Check sheet for the modelled part. Datum: model origin and axes. Units: mm. A direction names the side the tool comes from. Give positions to 0.01 mm unless a question says otherwise; leave off trailing zeros. Loops run counter-clockwise (first coordinate to the right, second up) from the corner with the lowest first, then second, coordinate; pieces in that order, holes last. Notation, with made-up numbers: (-25.5, -4.5) - (-11.5, -4.5) arc R18 cw to (-11.5, 28.5) - close; hole circle Ø4 at (87.5, 11.5). An arc over 180 degrees is marked (long way). Use one line per item in the form item = value.
from build123d import *

# Parameters (mm, degrees)
F0_W     = 714.670822
F0_H     = 1041.4
F1_DEPTH = 1397
F2_DEPTH = 1143
F0_W_2   = 127
F0_H_2   = 660.4
F3_DEPTH = 1092.2
F4_W     = 596.427142
F4_H     = 931.297839
F5_DEPTH = 873.76


with BuildPart() as f1:
    # F0 (on Top) → F1 (new body)
    with BuildSketch(Plane.XY):
        with Locations((988.864589, 12.7)):
            Rectangle(F0_W, F0_H)
    extrude(amount=F1_DEPTH)

    # F0 (on Top) → F2 (join)
    with BuildSketch(Plane.XY):
        Polygon((-203.2, 0), (0, 0), (0, -508), (631.529178, -508), (631.529178, 533.4), (799.153613, 903.620216), (58.713181, 1238.869088), (-203.2, 660.4), align=None)
    extrude(amount=F2_DEPTH)

    # F0 (on Top) → F3 (join)
    with BuildSketch(Plane.XY):
        with Locations((-266.7, 330.2)):
            Rectangle(F0_W_2, F0_H_2)
    extrude(amount=F3_DEPTH)

    # F4 (on face) → F5 (cut)
    with BuildSketch(Plane.XY.offset(1397)):
        with Locations((996.125251, 10.54573)):
            Rectangle(F4_W, F4_H)
    extrude(amount=-F5_DEPTH, mode=Mode.SUBTRACT)


solid = f1.part
Item 1: Section check C-C on y = 161.5. Record the boundary of the cut face in (x, z).
Answer block:
outline = (-330.2, 0) - (1346.2, 0) - (1346.2, 1397) - (1294.34, 1397) - (1294.34, 523.24) - (697.91, 523.24) - (697.91, 1397) - (631.53, 1397) - (631.53, 1143) - (-203.2, 1143) - (-203.2, 1092.2) - (-330.2, 1092.2) - close
Item 2: Section check A-A on z = 1206. Record the boundary of the cut face in (x, y), then the cut area to 3 significant figures.
Answer block:
outline = (631.53, -508) - (1346.2, -508) - (1346.2, 533.4) - (631.53, 533.4) - close; hole (697.91, -455.1) - (1294.34, -455.1) - (1294.34, 476.19) - (697.91, 476.19) - close
area = 189,000 mm2
Item 3: Access from +Z, -Z, +X, -X, +Y, -Y to the whole of each face (thin tool, end or side, straight path). Record for faces 1 (the face through (714.17, 715.92, 563.5)), 2 (the face through (992, -455.103, 966)), 3 (the face through (0, -250, 563)), 4 (the face through (434.116, 1068.898, 563.499)), 5 (the face through (-268, 335, 1092.2)).
Answer block:
face_1 = +Z, -Z, +X
face_2 = +Z
face_3 = +Z, -Z, -X, -Y
face_4 = +Z, -Z, +X, +Y
face_5 = +Z, -X, +Y, -Y
Item 4: Gauge pin test, flat ends, axial feed: P1, Ø4, axis at x = 895.5, y = -204.5, coming from the +Z side; P2, Ø8, axis at y = 1028.5, z = 668.5, coming from the -X side; P3, Ø2, axis at y = -60.5, z = 962, coming from the -X side. Record the tip position at first contact, or that the pin passes through.
Answer block:
P1 = 523.24
P2 = -38.35
P3 = 0
Item 5: Section check D-D on x = 914.5. Record the boundary of the cut face in (y, z).
Answer block:
outline = (-508, 0) - (533.4, 0) - (533.4, 1397) - (476.19, 1397) - (476.19, 523.24) - (-455.1, 523.24) - (-455.1, 1397) - (-508, 1397) - close
Item 6: Thickness scan on L1, parallel to X at y = 219.5, z = 789.5; L2, parallel to Y at x = 965.5, z = 1250.5; L3, parallel to X at y = -324, z = 1063.5. Record the ranges inside material, lowest first.
Answer block:
L1 = -330.2 to 697.91, 1294.34 to 1346.2
L2 = -508 to -455.1, 476.19 to 533.4
L3 = 0 to 697.91, 1294.34 to 1346.2
Item 7: Section check B-B on x = 661. Record the boundary of the cut face in (y, z), then the cut area to 3 significant figures.
Answer block:
outline = (-508, 0) - (533.4, 0) - (533.4, 1397) - (-508, 1397) - close; (598.49, 0) - (966.17, 0) - (966.17, 1143) - (598.49, 1143) - close
area = 1,880,000 mm2
Item 8: Mould release check, pull along Y, two halves, no side actions. Record for faces 6 (the face through (-203.2, 335, 1117)), 7 (the face through (-268, 660.4, 538)), 8 (the face through (697.912, 4, 966)), 9 (the face through (992, 476.195, 966)): released by +Y, released by -Y, zero draft, split by the parting line, or undercut.
Answer block:
face_6 = zero draft
face_7 = released by +Y
face_8 = undercut
face_9 = undercut
